Geometry: final body of the model. Coordinates: model frame, mm. Face numbers are marked on the shaded views. A direction names the side the tool comes from. Give positions to 0.01 mm unless a question says otherwise; leave off trailing zeros. Write each loop counter-clockwise with the first axis right and the second up, starting at its lowest first coordinate (ties: lowest second). Pieces come first, ordered by that corner, then holes.
from build123d import *

# Parameters (mm, degrees)
BOSS_EXTRUDE1_DEPTH = 530
SKETCH2_R           = 22.5
CUT_EXTRUDE1_DEPTH  = 530
SKETCH3_W           = 70
SKETCH3_H           = 59
CUT_EXTRUDE2_DEPTH  = 530


with BuildPart() as part:
    # Sketch1 → Boss-Extrude1 (new body)
    with BuildSketch(Plane.XY):
        Polygon((0, 0), (0, 530), (-0.35, 530), (-0.35, 0.35), (-30.35, 0.35), (-30.35, 0), align=None)
    extrude(amount=BOSS_EXTRUDE1_DEPTH)

    # Sketch2 → Cut-Extrude1 (cut)
    with BuildSketch(Plane.ZY.offset(0.35)):
        with Locations((170, 165.35)):
            Circle(SKETCH2_R)
    extrude(amount=-CUT_EXTRUDE1_DEPTH, mode=Mode.SUBTRACT)

    # Sketch3 → Cut-Extrude2 (cut)
    with BuildSketch(Plane.ZY.offset(0.35)):
        with Locations((335, 30.85)):
            Rectangle(SKETCH3_W, SKETCH3_H)
    extrude(amount=-CUT_EXTRUDE2_DEPTH, mode=Mode.SUBTRACT)


solid = part.part
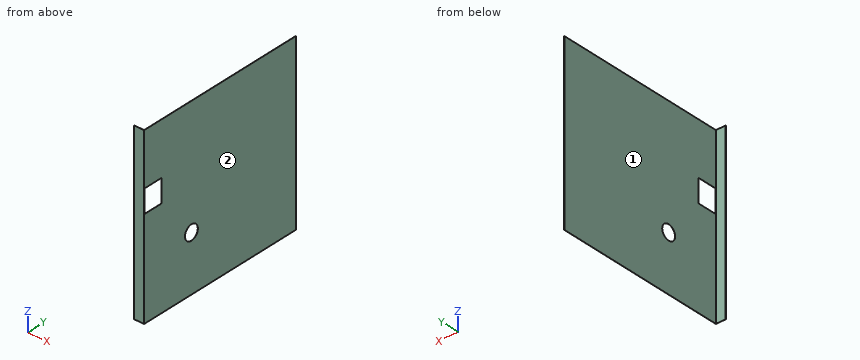
Q1. Section A-A on y = 165.35. Output: boundary loops of the cut face in (x, z).
Filled sheet:
outline: (-0.35, 0) - (0, 0) - (0, 147.5) - (-0.35, 147.5) - close; (-0.35, 192.5) - (0, 192.5) - (0, 530) - (-0.35, 530) - close
Q2. Section B-B on z = 323. Output: boundary loops of the cut face in (x, y).
Filled sheet:
outline: (-30.35, 0) - (0, 0) - (0, 1.35) - (-0.35, 1.35) - (-0.35, 0.35) - (-30.35, 0.35) - close; (-0.35, 60.35) - (0, 60.35) - (0, 530) - (-0.35, 530) - close
Q3. Section D-D on z = 170. Output: boundary loops of the cut face in (x, y), plus the area to 3 significant figures.
Filled sheet:
outline: (-30.35, 0) - (0, 0) - (0, 142.85) - (-0.35, 142.85) - (-0.35, 0.35) - (-30.35, 0.35) - close; (-0.35, 187.85) - (0, 187.85) - (0, 530) - (-0.35, 530) - close
area: 180 mm2
Q4. Access query for the marked faces 1 and 2. Directions: +Z, -Z, +X, -X, +Y, -Y. A direction counts if a zero-diameter tool reaches every point of the face in a straight line with its end or side. Return the directions, or none.
Filled sheet:
face 1: +Z, -Z, -X, +Y
face 2: +Z, -Z, +X, +Y, -Y
Q5. Section C-C on x = -24.5. Output: boundary loops of the cut face in (y, z), plus the area to 4 significant figures.
Filled sheet:
outline: (0, 0) - (0.35, 0) - (0.35, 530) - (0, 530) - close
area: 185.5 mm2
Q6. Pin query (flat end, axial travel): P1, Ø10, axis at y = 184, z = 362, coming from the -X side; P2, Ø2, axis at x = -21.5, z = 332, coming from the +Y side. Return the tip coordinate at first contact, or that it passes through.
Filled sheet:
P1: stops at x = -0.35
P2: stops at y = 0.35
Q7. Ray query, line 1 along Y through (x, z) = (-0.05, 170); line 2 along Y through (x, z) = (-14, 488.5); line 3 along X through (y, z) = (96, 83). Return the intervals inside material, ascending.
Filled sheet:
line 1: y = 0 to 142.85, 187.85 to 530
line 2: y = 0 to 0.35
line 3: x = -0.35 to 0
